Geometry check sheet. Reference: drawing and pictorial views, mm from the part's lowest x, y, z. A direction names the side the tool comes from. Give positions to 0.01 mm unless a question says otherwise; leave off trailing zeros. Loops run counter-clockwise (first coordinate to the right, second up) from the corner with the lowest first, then second, coordinate; pieces in that order, holes last. Notation, with made-up numbers: (83.5, 10.5) - (130.5, 10.5) arc R26 ccw to (130.5, 49.5) - close; hole circle Ø1 at (80, 76.5). An arc over 180 degrees is marked (long way). One line per question, with ' | ' between items. Start each with the question number.
1. Mould release check, pull along X, two halves, no side actions. Record for the marked faces 3, 4, 5 and 6: +X half, -X half, draft (parallel to the pull), parting line (faces both ways), or undercut.
2. Section check A-A, the plane z = 26. Enter the section's corners in (x, y) (3 decimals), then the cut area to 3 significant figures.
3. Section check C-C, the plane x = 13.5. Enter the section's corners in (y, z).
4. Thickness scan on line 1 along Z through (x, y) = (8.5, 22); line 2 along X through (y, z) = (12, 14); line 3 along X through (y, z) = (3, 9). Record the ranges inside material, lowest first. Write a range as from..to.
5. Tool access check on the marked faces 1 and 2. Record the directions out of +Z, -Z, +X, -X, +Y, -Y that give a thin tool (end or side, any length) a straight path to the whole face; none if there is none.
6. Section check B-B, the plane y = 5.75. Enter the section's corners in (x, z).
7. Depth check by flat-ended pin: pin 1 Ø8 at (x, y) = (14.5, 18.5) entering from -Z; pin 2 Ø3.5 at (x, z) = (8.5, 12) entering from -Y (3 decimals). Enter the tip coordinate at first touch or a pass-through.
8. Section check D-D, the plane z = 5.5. Enter the section's corners in (x, y), then the cut area to 3 significant figures.
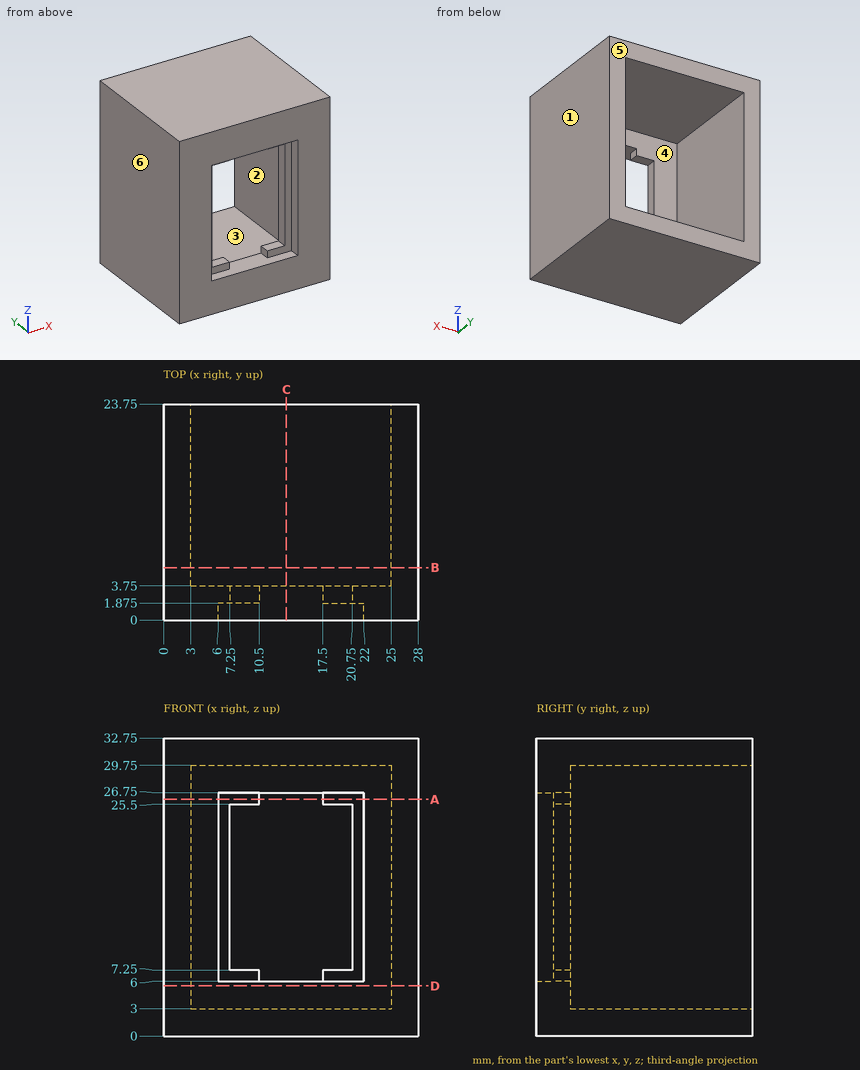
Results list:
1) face 3: undercut | face 4: undercut | face 5: draft | face 6: -X half
2) outline: (0, 0) - (6, 0) - (6, 1.875) - (10.5, 1.875) - (10.5, 3.75) - (3, 3.75) - (3, 23.75) - (0, 23.75) - close; (17.5, 1.875) - (22, 1.875) - (22, 0) - (28, 0) - (28, 23.75) - (25, 23.75) - (25, 3.75) - (17.5, 3.75) - close | area: 182 mm²
3) outline: (0, 0) - (23.75, 0) - (23.75, 3) - (3.75, 3) - (3.75, 6) - (0, 6) - close; (0, 26.75) - (3.75, 26.75) - (3.75, 29.75) - (23.75, 29.75) - (23.75, 32.75) - (0, 32.75) - close
4) line 1: 0..3, 29.75..32.75 | line 2: 0..3, 25..28 | line 3: 0..7.25, 20.75..28
5) face 1: +Z, -Z, +X, +Y, -Y | face 2: +Y
6) outline: (0, 0) - (28, 0) - (28, 32.75) - (0, 32.75) - close; hole (3, 3) - (25, 3) - (25, 29.75) - (3, 29.75) - close
7) pin 1: z = 0 | pin 2: y = 1.875
8) outline: (0, 0) - (28, 0) - (28, 23.75) - (25, 23.75) - (25, 3.75) - (3, 3.75) - (3, 23.75) - (0, 23.75) - close | area: 225 mm²
